```python
from build123d import *

# Parameters (mm, degrees)
SKETCH3_R           = 7.5
BOSS_EXTRUDE2_DEPTH = 17
SKETCH5_R           = 1
CUT_EXTRUDE1_DEPTH  = 17
FILLET5_R           = 2
FILLET6_R           = 2


with BuildPart() as part:
    # Sketch3 → Boss-Extrude2 (new body)
    with BuildSketch(Plane.XY):
        Circle(SKETCH3_R)
    extrude(amount=BOSS_EXTRUDE2_DEPTH)

    # Sketch5 → Cut-Extrude1 (cut)
    with BuildSketch(Plane.XY.offset(17)):
        Circle(SKETCH5_R)
    extrude(amount=-CUT_EXTRUDE1_DEPTH, mode=Mode.SUBTRACT)

    # Fillet5
    fillet5_edges = [part.edges().sort_by_distance(p)[0] for p in [
        (-7.5, 0, 17),
    ]]
    fillet(fillet5_edges, radius=FILLET5_R)

    # Fillet6
    fillet6_edges = [part.edges().sort_by_distance(p)[0] for p in [
        (-7.5, 0, 0),
    ]]
    fillet(fillet6_edges, radius=FILLET6_R)


solid = part.part
```
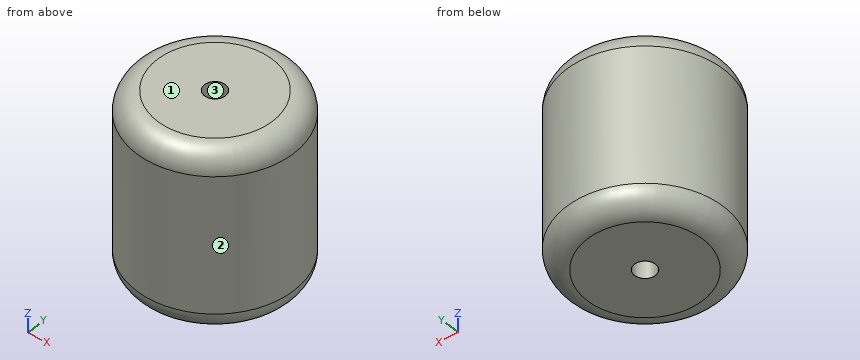
Input: part model. Units: mm. Frame: model coordinates. Face numbers are marked on the shaded views. Coordinates: 2 decimals unless noted, no trailing zeros. Write each loop counter-clockwise with the first axis right and the second up, starting at its lowest first coordinate (ties: lowest second). Pieces come first, ordered by that corner, then holes. Notation, with made-up numbers: (67.25, -33.5) - (94.25, -33.5) arc R21 ccw to (94.25, -17.5) - close; hole circle Ø7 at (8.5, 83). An arc over 180 degrees is marked (long way). Put each result on its own line as item: value. Start each with the question number.
1) Cut plane A-A (x = 0). Return the cut outline in (y, z).
2) Cut plane C-C (z = 9.25). Return the cut outline in (x, y).
3) Mould query, pull axis X, two halves, no side actions, for the marked faces 1, 2 and 3. Classes: pulls with the +X half, pulls with the -X half, needs draft (parallel to the pull), parting line crosses it, or undercut.
4) Contact query for flat-ended pins moving along their axis: pin 1 (5 mm diameter, centred on x = 0.5, y = -1, fed in from -Z); pin 2 (6 mm diameter, centred on x = -5.5, z = 8.5, fed in from -Y); pin 3 (3 mm diameter, centred on y = 2, z = 8.5, fed in from -X); pin 4 (6 mm diameter, centred on y = -5.5, z = 1.5, fed in from -X). Output: stop coordinate, or through.
5) Ray query, L1, parallel to Y at x = 0, z = 12.25; L2, parallel to Z at x = 5.5, y = 1.25; L3, parallel to Z at x = 2.25, y = -6. Return the intervals inside material, ascending.
Resolved:
1. outline: (-7.5, 2) arc R2 ccw to (-5.5, 0) - (-1, 0) - (-1, 17) - (-5.5, 17) arc R2 ccw to (-7.5, 15) - close; (1, 0) - (5.5, 0) arc R2 ccw to (7.5, 2) - (7.5, 15) arc R2 ccw to (5.5, 17) - (1, 17) - close
2. outline: circle Ø15 at (0, 0); hole circle Ø2 at (0, 0)
3. face 1: needs draft
3. face 2: parting line crosses it
3. face 3: undercut
4. pin 1: stops at z = 0
4. pin 2: stops at y = -7.07
4. pin 3: stops at x = -7.48
4. pin 4: stops at x = -7.06
5. L1: y = -7.5 to -1, 1 to 7.5
5. L2: z = 0 to 17
5. L3: z = 0.22 to 16.78
